Input: part model. Units: mm. Frame: model coordinates. A direction names the side the tool comes from. Coordinates: 2 decimals unless noted, no trailing zeros. Loops run counter-clockwise (first coordinate to the right, second up) from the corner with the lowest first, then second, coordinate; pieces in that order, holes last. Notation, with made-up numbers: (-30, 2.25) -> (-8, 2.25) arc R21 ccw to (-8, 18.25) -> close; hole circle Ø11 at (-20, 70.25). An arc over 180 degrees is marked (long way). Put each result on its own line as item: value. Start each with the question number.
1) Cut plane A-A (y = 15). State how many separate pieces and enclosed holes the cut face has, plus the area to 3 significant figures.
2) Cut plane B-B (z = 23.5). Return the cut outline in (x, y).
3) Pull-direction query (Z, two-part tool) for faces 3 (the conical face through (11.41, -2.53, 117.71)), 4 (the flat face through (0, 0, 124)), 5 (the cylindrical face through (-21.477, -4.769, 122.409)); classes: pulls with the +Z half, pulls with the -Z half, needs draft (parallel to the pull), parting line crosses it, or undercut.
4) Material intervals for L1, parallel to Y at x = -0.5, z = 19.5; L2, parallel to X at y = 4, z = 111; L3, parallel to X at y = -8, z = 104.5, sorted ascending.
5) Set-up query: faces 1 (the cylindrical face through (-21.477, -4.769, 97.984)), 2 (the cylindrical face through (-10.74, -2.38, 67.98)). Return all of +Z, -Z, +X, -X, +Y, -Y with unobstructed straight access to the full face (end or side cutting, diameter ignored); none if empty.
6) Contact query for flat-ended pins moving along their axis: P1, Ø6, axis at x = -9.5, z = 26, coming from the -Y side; P2, Ø5, axis at y = 11.5, z = 13.5, coming from the +X side; P3, Ø3, axis at x = 13.5, z = 86.5, coming from the +Y side; P4, Ø1.5, axis at x = 17.5, z = 78.5, coming from the +Y side. Output: stop coordinate, or through.
Autodesk Inventor part; units mm, degrees
ref_plane "Belt Plane" through (0, 11, 8) normal (0, 0, 1) x (1, 0, 0)
ref_plane "YZ Plane" through (0, 0, 0) normal (1, 0, 0) x (0, 1, 0)
ref_plane "XZ Plane" through (0, 0, 0) normal (0, 1, 0) x (-1, 0, 0)
sketch "Main Sketch" plane through (0, 0, 0) normal (1, 0, 0) x (0, 1, 0)
  line L0 (0, 124) -> (22, 124)
  line L1 (22, 124) -> (22, 12.8615)
  line L2 (22, 12.8615) -> (11, 9.4984)
  line L3 (11, 9.4984) -> (11, 6.5016)
  line L4 (11, 6.5016) -> (22, 3.1385)
  line L5 (22, 3.1385) -> (22, 0)
  line L6 (22, 0) -> (0, 0)
  line L7 (20, 12.25) -> (20, 3.75) construction
  line L8 (11, 8) -> (20, 8) construction
  line L9 (22, 12.8615) -> (22, 3.1385)
  line L10 (0, -4) -> (0, 24)
  line L11 (0, 0) -> (0, 124)
  dimension "d0" = 8.5
  dimension "d1" = 34
  dimension "d2" = 2
  dimension "d6" = 124
  dimension "d21" = 40
  dimension "d25" = 11
  dimension "d27" = 8
ref_plane "Belt Plane" through (0, 11, 8) normal (0, 0, 1) x (1, 0, 0)
revolve "Body" add sketch "Main Sketch" angle 360 about axis through (0, 0, -10) along (0, 0, 1)
revolve "Groove" cut sketch "Main Sketch" angle 360 about axis through (0, 0, -10) along (0, 0, 1) contours L9 L4 L3 L2
fillet "Fillet External" [suppressed]
fillet "Fillet Internal" [suppressed]
pattern_linear "Groove Pattern" count 10 spacing 12 along (0, 0, 1) of "Groove"
equation "\"d0\" = da_Bw"
equation "\"d1\" = da_Alfa"
equation "\"d2\" = da_c"
equation "\"d21\" = da_Dw"
equation "\"d25\" = da_Hd"
equation "\"d27\" = da_Se"
equation "\"da_r1\" = 0"
equation "\"da_r2\" = 0"
equation "\"d18\" = da_Sg"
equation "\"d5\" = da_Se"
equation "\"da_Bw\" = 8.5"
equation "\"da_Alfa\" = 34deg"
equation "\"da_c\" = 2"
equation "\"da_Dw\" = 40"
equation "\"da_Hd\" = 11"
equation "\"da_Se\" = 8"
equation "\"da_Sg\" = 12"
properties part number "Grooved Pulley1" material "Steel"
Results found:
1. separate pieces: 11
1. enclosed holes: 0
1. area: 1,740 mm2
2. outline: circle Ø35.09 at (0, 0)
3. face 3: undercut
3. face 4: pulls with the +Z half
3. face 5: needs draft
4. L1: y = -10.99 to 10.99
4. L2: x = -21.63 to 21.63
4. L3: x = -7.55 to 7.55
5. face 1: +Z, -Z
5. face 2: none
6. P1: stops at y = -21.02
6. P2: stops at x = 20.07
6. P3: stops at y = 18.44
6. P4: passes through
